Work out the finished part from the listing and answer in its coordinate system (mm). Coordinates: 2 decimals unless noted, no trailing zeros. Loops run counter-clockwise (first coordinate to the right, second up) from the corner with the lowest first, then second, coordinate; pieces in that order, holes last. Notation, with made-up numbers: (20.5, 8.5) -> (30.5, 8.5) arc R12 ccw to (30.5, 25.5) -> close; hole circle Ø3 at (49.25, 82.5). An arc over 180 degrees is marked (long way). Use a Markdown table: item, result.
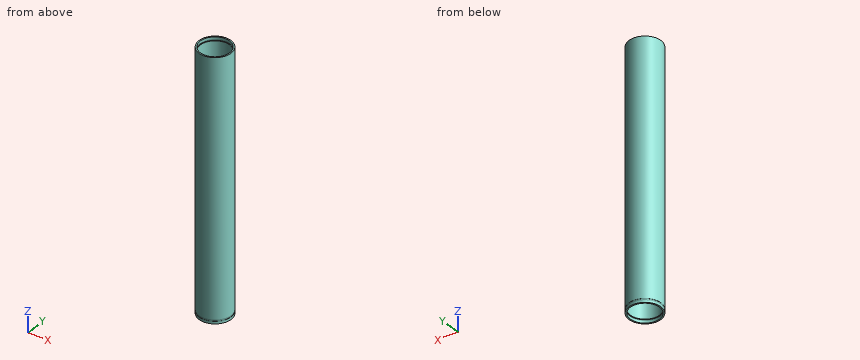
Autodesk Inventor part; units mm, degrees
ref_plane "Work Plane1" through (0, 0, 192) normal (0, 0, 1) x (1, 0, 0)
ref_plane "Work Plane2" through (0, 0, 3.8) normal (0, 0, -1) x (-1, 0, 0)
ref_plane "YZ Plane" through (0, 0, 0) normal (1, 0, 0) x (0, 1, 0)
sketch "Sketch1" plane through (0, 0, 0) normal (0, 0, 1) x (1, 0, 0)
  circle A0 centre (0, 0) radius 24
  circle A1 centre (0, 0) radius 22
  dimension "d0" = 48
  dimension "d1" = 44
extrude "Extrusion1" add sketch "Sketch1" along normal blind 384
ref_plane "Work Plane1" through (0, 0, 192) normal (0, 0, 1) x (1, 0, 0)
ref_plane "Work Plane2" through (0, 0, 3.8) normal (0, 0, -1) x (-1, 0, 0)
sketch "Sketch2" plane through (0, 0, 0) normal (0, 0, -1) x (-1, 0, 0)
  circle A0 centre (0, 0) radius 23.25
  circle A1 centre (0, 0) radius 22
  dimension "d4" = 46.5
extrude "Extrusion2" cut sketch "Sketch2" against normal blind 1.85 from surface at -3.8
mirror "Mirror1" about plane through (0, 0, 192) normal (0, 0, 1) of "Extrusion2"
sketch "Sketch3" plane through (0, 0, 0) normal (0, 0, -1) x (-1, 0, 0)
  circle A0 centre (0, 0) radius 23.75
  circle A1 centre (0, 0) radius 24
  dimension "d8" = 47.5
extrude "Extrusion3" cut sketch "Sketch3" against normal up to surface (1.85 mm away) from surface at -3.8
properties part number "SRM 2020 Casing EE5" material "Aluminum 6061"
Q1. Section C-C on z = 29.5 is taken. Determine the outline of the cut face in (x, y), and give its area (3 significant figures).
Solved:
| item | result |
|---|---|
| outline | circle Ø48 at (0, 0); hole circle Ø44 at (0, 0) |
| area | 289 mm² |
Q2. Given pin 1 Ø2 at (y, z) = (-10.5, 101) entering from +X; pin 2 Ø10 at (x, y) = (-14, 8) entering from -Z; pin 3 Ø2 at (y, z) = (-13.5, 216.5) entering from +X; pin 4 Ø3 at (y, z) = (-10.5, 243) entering from -X, each flat-ended and moving along its own axis, determine where each tip first touches the part or whether it passes through.
Solved:
| item | result |
|---|---|
| pin 1 | x = 22.04 |
| pin 2 | through |
| pin 3 | x = 20.49 |
| pin 4 | x = -22.25 |
Q3. Consider line 1 (Y direction, x = 0, z = 1.4); line 2 (Y direction, x = -14, z = 108). Determine where each line is inside the solid, lowest interval first. Write a range as [from, to].
Solved:
| item | result |
|---|---|
| line 1 | [-24, -22], [22, 24] |
| line 2 | [-19.49, -16.97], [16.97, 19.49] |
